Geometry check sheet. Reference: the model listing, model coordinates, mm. Face numbers are marked on the shaded views. A direction names the side the tool comes from. Coordinates: 2 decimals unless noted, no trailing zeros. Order: outer loops, then holes, each group sorted by start corner. A loop starts at its lowest first (then second) coordinate and runs counter-clockwise, first axis right, second up.
```python
from build123d import *

# Parameters (mm, degrees)
SKETCH1_R             = 29.75
BOSS_EXTRUDE1_DEPTH   = 16
SKETCH2_R             = 35.8
BOSS_EXTRUDE2_DEPTH   = 47.5
M4_TAPPED_HOLE1_D     = 3.3
M4_TAPPED_HOLE1_DEPTH = 6
M4_TAPPED_HOLE1_TIP   = 0.991420021
SKETCH6_R             = 6
CUT_EXTRUDE1_DEPTH    = 20
CHAMFER1_SIZE         = 1
CHAMFER2_SIZE         = 1
CHAMFER2_SIZE2        = 3.732050808
CUT_EXTRUDE2_START    = 20
SKETCH7_W             = 25
SKETCH7_H             = 13
CUT_EXTRUDE2_DEPTH    = 20


with BuildPart() as part:
    # Sketch1 → Boss-Extrude1 (new body)
    with BuildSketch(Plane(origin=(0, 0, 0), x_dir=(1, 0, 0), z_dir=(0, 1, 0))):
        Circle(SKETCH1_R)
    extrude(amount=BOSS_EXTRUDE1_DEPTH)

    # Sketch2 → Boss-Extrude2 (add)
    with BuildSketch(Plane(origin=(0, 16, 0), x_dir=(1, 0, 0), z_dir=(0, 1, 0))):
        Circle(SKETCH2_R)
    extrude(amount=BOSS_EXTRUDE2_DEPTH)

    # M4 Tapped Hole1
    with Locations(Plane(origin=(0, 63.5, 0), x_dir=(1, 0, 0), z_dir=(0, 1, 0))):
        with Locations((0, 20), (17.320508076, -10), (-17.320508076, -10)):
            Hole(M4_TAPPED_HOLE1_D / 2, depth=M4_TAPPED_HOLE1_DEPTH)
            with Locations((0, 0, -(M4_TAPPED_HOLE1_DEPTH + M4_TAPPED_HOLE1_TIP / 2))):  # 118° drill point
                Cone(0, M4_TAPPED_HOLE1_D / 2, M4_TAPPED_HOLE1_TIP, mode=Mode.SUBTRACT)

    # Sketch6 → Cut-Extrude1 (cut)
    with BuildSketch(Plane(origin=(0, 63.5, 0), x_dir=(1, 0, 0), z_dir=(0, 1, 0))):
        Circle(SKETCH6_R)
    extrude(amount=-CUT_EXTRUDE1_DEPTH, mode=Mode.SUBTRACT)

    # Chamfer1
    chamfer1_edges = [part.edges().sort_by_distance(p)[0] for p in [
        (-35.8, 63.5, 0),
    ]]
    chamfer(chamfer1_edges, length=CHAMFER1_SIZE)

    # Chamfer2
    chamfer2_edges = [part.edges().sort_by_distance(p)[0] for p in [
        (-29.75, 0, 0),
    ]]
    chamfer2_side = [part.faces().sort_by_distance(p)[0] for p in [
        (-29.75, 8, 0),
    ]]
    chamfer(chamfer2_edges, length=CHAMFER2_SIZE, length2=CHAMFER2_SIZE2, reference=chamfer2_side[0])

    # Sketch7 → Cut-Extrude2 (cut)
    with BuildSketch(Plane.XY.offset(CUT_EXTRUDE2_START)):
        with Locations((0, 9.5)):
            Rectangle(SKETCH7_W, SKETCH7_H)
    extrude(amount=CUT_EXTRUDE2_DEPTH, mode=Mode.SUBTRACT)


solid = part.part
```
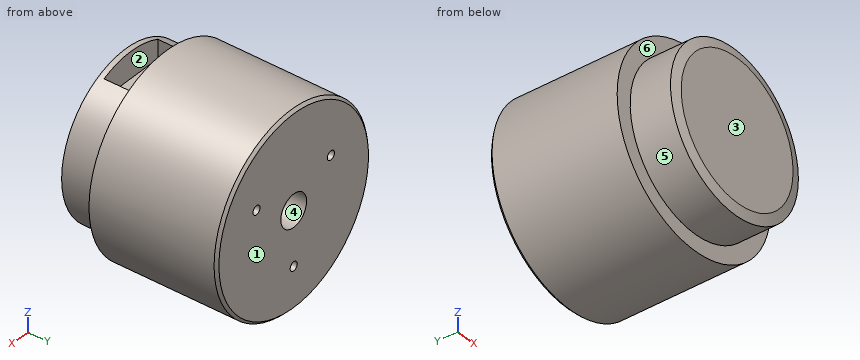
Item 1: Tool access check on the marked faces 1 and 2. Record the directions out of +Z, -Z, +X, -X, +Y, -Y that give a thin tool (end or side, any length) a straight path to the whole face; none if there is none.
Item 2: Depth check by flat-ended pin: P1, Ø10, axis at y = 28, z = 17.5, coming from the -X side; P2, Ø3, axis at x = -22, y = 41, coming from the -Z side; P3, Ø3, axis at y = 35.5, z = -27.5, coming from the +X side. Enter the tip coordinate at first touch or a pass-through.
Item 3: Sectioned sample at C-C (y = 9). Record the cut outline in (x, z).
Item 4: Release check for a two-part mould opening along X. For the marked faces 3, 4, 5 and 6 record: pulls with the +X half, pulls with the -X half, needs draft (parallel to the pull), parting line crosses it, or undercut.
Item 5: Thickness scan on line 1 along Z through (x, y) = (0, 57.5); line 2 along X through (y, z) = (61.8, 10) (1 decimal); line 3 along X through (y, z) = (50.5, 0). Record the ranges inside material, lowest first.
Item 6: Sectioned sample at A-A (z = 0). Record the cut outline in (x, y), and give its area (3 significant figures).
Item 7: Sectioned sample at B-B (y = 58.5). Record the cut outline in (x, z).
Geometry check:
1. face 1: +Z, -Z, +X, -X, +Y
1. face 2: +Z
2. P1: stops at x = -33.55
2. P2: stops at z = -29.35
2. P3: stops at x = 24.61
3. outline: (-12.5, 20) - (-12.5, 27) arc R29.75 ccw (long way) to (12.5, 27) - (12.5, 20) - close
4. face 3: needs draft
4. face 4: undercut
4. face 5: parting line crosses it
4. face 6: undercut
5. line 1: z = -35.8 to -21.65, -18.35 to -6, 6 to 35.8
5. line 2: x = -34.4 to -19, -15.7 to 15.7, 19 to 34.4
5. line 3: x = -35.8 to -6, 6 to 35.8
6. outline: (-35.8, 16) - (-29.75, 16) - (-29.75, 1) - (-26.02, 0) - (26.02, 0) - (29.75, 1) - (29.75, 16) - (35.8, 16) - (35.8, 62.5) - (34.8, 63.5) - (6, 63.5) - (6, 43.5) - (-6, 43.5) - (-6, 63.5) - (-34.8, 63.5) - (-35.8, 62.5) - close
6. area: 4,110 mm2
7. outline: circle Ø71.6 at (0, 0); hole circle Ø3.3 at (-17.32, 10); hole circle Ø12 at (0, 0); hole circle Ø3.3 at (0, -20); hole circle Ø3.3 at (17.32, 10)
